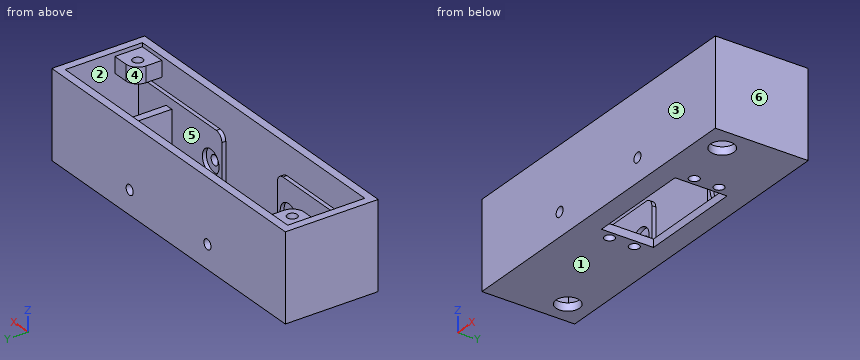
```python
from build123d import *

# Parameters (mm, degrees)
SKETCH1_W                      = 127
SKETCH1_H                      = 31.115
BOSS_EXTRUDE1_DEPTH            = 3.175
CUT_EXTRUDE1_REACH             = 5.175
SKETCH2_R                      = 2
SKETCH2_W                      = 42
SKETCH2_H                      = 21
SKETCH3_W                      = 133.35
SKETCH3_H                      = 37.465
SKETCH3_W_2                    = 127
SKETCH3_H_2                    = 31.115
EXTRUDE_THIN1_DEPTH            = 31.75
EXTRUDE_THIN1_DEPTH_BACK       = 3.175
SKETCH4_W                      = 47.625
SKETCH4_H                      = 1.5875
BOSS_EXTRUDE2_DEPTH            = 19.67500002
CUT_EXTRUDE2_REACH             = 5.175
SKETCH6_R                      = 4.7625
BOSS_EXTRUDE4_START            = -1.5875
BOSS_EXTRUDE4_DEPTH            = 6.35
CUT_EXTRUDE3_REACH             = 36.925
SKETCH8_R                      = 2
SKETCH9_R                      = 2
CUT_EXTRUDE4_DEPTH             = 19.7325
CUT_EXTRUDE4_DEPTH_BACK        = 19.7325
SKETCH5_W                      = 3.175
SKETCH5_H                      = 27.94
BOSS_EXTRUDE3_DEPTH            = 15.875
FILLET1_R                      = 3.175
CUT_EXTRUDE5_REACH             = 20.733
SKETCH10_R                     = 4.7625
CUT_EXTRUDE5_DIRECTION_2_REACH = 20.733


with BuildPart() as part:
    # Sketch1 → Boss-Extrude1 (new body)
    with BuildSketch(Plane.XY):
        Rectangle(SKETCH1_W, SKETCH1_H)
    extrude(amount=BOSS_EXTRUDE1_DEPTH)

    # Sketch2 → Cut-Extrude1 (cut, up to next)
    with BuildSketch(Plane.XY.offset(3.175), mode=Mode.PRIVATE) as cut_extrude1_sk1:
        with Locations((-13.2, 5)):
            Circle(SKETCH2_R)
    cut_extrude1_tool1 = extrude(cut_extrude1_sk1.sketch, amount=-CUT_EXTRUDE1_REACH, mode=Mode.PRIVATE) & part.part
    add(cut_extrude1_tool1.solids().sort_by_distance((-13.2, 5, 3.175))[0], mode=Mode.SUBTRACT)
    # Sketch2 → Cut-Extrude1 (cut, up to next)
    with BuildSketch(Plane.XY.offset(3.175), mode=Mode.PRIVATE) as cut_extrude1_sk2:
        with Locations((-13.2, -5)):
            Circle(SKETCH2_R)
    cut_extrude1_tool2 = extrude(cut_extrude1_sk2.sketch, amount=-CUT_EXTRUDE1_REACH, mode=Mode.PRIVATE) & part.part
    add(cut_extrude1_tool2.solids().sort_by_distance((-13.2, -5, 3.175))[0], mode=Mode.SUBTRACT)
    # Sketch2 → Cut-Extrude1 (cut, up to next)
    with BuildSketch(Plane.XY.offset(3.175), mode=Mode.PRIVATE) as cut_extrude1_sk3:
        with Locations((35.2, 5)):
            Circle(SKETCH2_R)
    cut_extrude1_tool3 = extrude(cut_extrude1_sk3.sketch, amount=-CUT_EXTRUDE1_REACH, mode=Mode.PRIVATE) & part.part
    add(cut_extrude1_tool3.solids().sort_by_distance((35.2, 5, 3.175))[0], mode=Mode.SUBTRACT)
    # Sketch2 → Cut-Extrude1 (cut, up to next)
    with BuildSketch(Plane.XY.offset(3.175), mode=Mode.PRIVATE) as cut_extrude1_sk4:
        with Locations((35.2, -5)):
            Circle(SKETCH2_R)
    cut_extrude1_tool4 = extrude(cut_extrude1_sk4.sketch, amount=-CUT_EXTRUDE1_REACH, mode=Mode.PRIVATE) & part.part
    add(cut_extrude1_tool4.solids().sort_by_distance((35.2, -5, 3.175))[0], mode=Mode.SUBTRACT)
    # Sketch2 → Cut-Extrude1 (cut, up to next)
    with BuildSketch(Plane.XY.offset(3.175), mode=Mode.PRIVATE) as cut_extrude1_sk5:
        with Locations((11, 0)):
            Rectangle(SKETCH2_W, SKETCH2_H)
    cut_extrude1_tool5 = extrude(cut_extrude1_sk5.sketch, amount=-CUT_EXTRUDE1_REACH, mode=Mode.PRIVATE) & part.part
    add(cut_extrude1_tool5.solids().sort_by_distance((11, 0, 3.175))[0], mode=Mode.SUBTRACT)

    # Sketch3 → Extrude-Thin1 (add, two sides)
    with BuildSketch(Plane.XY.offset(3.175)) as extrude_thin1_sk:
        Rectangle(SKETCH3_W, SKETCH3_H)
        Rectangle(SKETCH3_W_2, SKETCH3_H_2, mode=Mode.SUBTRACT)
    extrude(amount=EXTRUDE_THIN1_DEPTH)
    extrude(extrude_thin1_sk.sketch, amount=-EXTRUDE_THIN1_DEPTH_BACK)

    # Sketch4 → Boss-Extrude2 (add)
    with BuildSketch(Plane.XY.offset(3.175)):
        with Locations((-39.6875, -14.76375)):
            Rectangle(SKETCH4_W, SKETCH4_H)
        with Locations((39.6875, -14.76375)):
            Rectangle(SKETCH4_W, SKETCH4_H)
        with Locations((-39.6875, 14.76375)):
            Rectangle(SKETCH4_W, SKETCH4_H)
        with Locations((39.6875, 14.76375)):
            Rectangle(SKETCH4_W, SKETCH4_H)
    extrude(amount=BOSS_EXTRUDE2_DEPTH)

    # Sketch6 → Cut-Extrude2 (cut, up to next)
    with BuildSketch(Plane.XY.offset(3.175), mode=Mode.PRIVATE) as cut_extrude2_sk1:
        with Locations((-57.15, 9.2075)):
            Circle(SKETCH6_R)
    cut_extrude2_tool1 = extrude(cut_extrude2_sk1.sketch, amount=-CUT_EXTRUDE2_REACH, mode=Mode.PRIVATE) & part.part
    add(cut_extrude2_tool1.solids().sort_by_distance((-57.15, 9.2075, 3.175))[0], mode=Mode.SUBTRACT)
    # Sketch6 → Cut-Extrude2 (cut, up to next)
    with BuildSketch(Plane.XY.offset(3.175), mode=Mode.PRIVATE) as cut_extrude2_sk2:
        with Locations((57.15, -9.2075)):
            Circle(SKETCH6_R)
    cut_extrude2_tool2 = extrude(cut_extrude2_sk2.sketch, amount=-CUT_EXTRUDE2_REACH, mode=Mode.PRIVATE) & part.part
    add(cut_extrude2_tool2.solids().sort_by_distance((57.15, -9.2075, 3.175))[0], mode=Mode.SUBTRACT)

    # Sketch7 → Boss-Extrude4 (add)
    with BuildSketch(Plane.XY.offset(34.925).offset(BOSS_EXTRUDE4_START)):
        with BuildLine():
            Line((-63.5, 15.5575), (-63.5, 4.445))
            Line((-63.5, 4.445), (-57.15, 4.445))
            ThreePointArc((-57.15, 4.445), (-53.782403955, 5.839903955), (-52.3875, 9.2075))
            Line((-52.3875, 9.2075), (-52.3875, 15.5575))
            Line((-52.3875, 15.5575), (-63.5, 15.5575))
        make_face()
        with BuildLine():
            Line((63.5, -15.5575), (52.3875, -15.5575))
            Line((52.3875, -15.5575), (52.3875, -9.2075))
            ThreePointArc((52.3875, -9.2075), (53.782403955, -5.839903955), (57.15, -4.445))
            Line((57.15, -4.445), (63.5, -4.445))
            Line((63.5, -4.445), (63.5, -15.5575))
        make_face()
    extrude(amount=-BOSS_EXTRUDE4_DEPTH)

    # Sketch8 → Cut-Extrude3 (cut, up to next)
    with BuildSketch(Plane.XY.offset(34.925), mode=Mode.PRIVATE) as cut_extrude3_sk1:
        with Locations((-57.15, 9.2075)):
            Circle(SKETCH8_R)
    cut_extrude3_tool1 = extrude(cut_extrude3_sk1.sketch, amount=-CUT_EXTRUDE3_REACH, mode=Mode.PRIVATE) & part.part
    add(cut_extrude3_tool1.solids().sort_by_distance((-57.15, 9.2075, 34.925))[0], mode=Mode.SUBTRACT)
    # Sketch8 → Cut-Extrude3 (cut, up to next)
    with BuildSketch(Plane.XY.offset(34.925), mode=Mode.PRIVATE) as cut_extrude3_sk2:
        with Locations((57.15, -9.2075)):
            Circle(SKETCH8_R)
    cut_extrude3_tool2 = extrude(cut_extrude3_sk2.sketch, amount=-CUT_EXTRUDE3_REACH, mode=Mode.PRIVATE) & part.part
    add(cut_extrude3_tool2.solids().sort_by_distance((57.15, -9.2075, 34.925))[0], mode=Mode.SUBTRACT)

    # Sketch9 → Cut-Extrude4 (cut, two sides)
    with BuildSketch(Plane(origin=(0, 0, 0), x_dir=(1, 0, 0), z_dir=(0, 1, 0))) as cut_extrude4_sk:
        with Locations((22.225, -9.525)):
            Circle(SKETCH9_R)
        with Locations((-22.225, -9.525)):
            Circle(SKETCH9_R)
    extrude(amount=CUT_EXTRUDE4_DEPTH, mode=Mode.SUBTRACT)
    extrude(cut_extrude4_sk.sketch, amount=-CUT_EXTRUDE4_DEPTH_BACK, mode=Mode.SUBTRACT)

    # Sketch5 → Boss-Extrude3 (add)
    with BuildSketch(Plane.XY.offset(3.175)):
        with Locations((46.0375, 0)):
            Rectangle(SKETCH5_W, SKETCH5_H)
        with Locations((-46.0375, 0)):
            Rectangle(SKETCH5_W, SKETCH5_H)
    extrude(amount=BOSS_EXTRUDE3_DEPTH)

    # Fillet1
    fillet1_edges = [part.edges().sort_by_distance(p)[0] for p in [
        (15.875, 14.76375, 22.85000002),
        (-15.875, -14.76375, 22.85000002),
        (15.875, -14.76375, 22.85000002),
        (-15.875, 14.76375, 22.85000002),
    ]]
    fillet(fillet1_edges, radius=FILLET1_R)

    # Cut-Extrude5: up to this face of the body (flat: up to its plane)
    cut_extrude5_end = Plane(part.part.faces().sort_by_distance((-1.954505757, -15.5575, 24.090116644))[0])
    # Sketch10 → Cut-Extrude5 (cut, up to the picked face)
    with BuildSketch(Plane(origin=(0, 0, 0), x_dir=(1, 0, 0), z_dir=(0, 1, 0)), mode=Mode.PRIVATE) as cut_extrude5_sk1:
        with Locations((-22.225, -9.525)):
            Circle(SKETCH10_R)
    cut_extrude5_tool1 = split(extrude(cut_extrude5_sk1.sketch, amount=-CUT_EXTRUDE5_REACH, mode=Mode.PRIVATE), bisect_by=cut_extrude5_end, keep=Keep.BOTH, mode=Mode.PRIVATE)
    add(cut_extrude5_tool1.solids().sort_by_distance((-22.225, 0, 9.525))[0], mode=Mode.SUBTRACT)
    # Sketch10 → Cut-Extrude5 (cut, up to the picked face)
    with BuildSketch(Plane(origin=(0, 0, 0), x_dir=(1, 0, 0), z_dir=(0, 1, 0)), mode=Mode.PRIVATE) as cut_extrude5_sk2:
        with Locations((22.225, -9.525)):
            Circle(SKETCH10_R)
    cut_extrude5_tool2 = split(extrude(cut_extrude5_sk2.sketch, amount=-CUT_EXTRUDE5_REACH, mode=Mode.PRIVATE), bisect_by=cut_extrude5_end, keep=Keep.BOTH, mode=Mode.PRIVATE)
    add(cut_extrude5_tool2.solids().sort_by_distance((22.225, 0, 9.525))[0], mode=Mode.SUBTRACT)

    # Cut-Extrude5 direction 2: up to this face of the body (flat: up to its plane)
    cut_extrude5_direction_2_end = Plane(part.part.faces().sort_by_distance((1.954505757, 15.5575, 24.090116644))[0])
    # Sketch10 → Cut-Extrude5 direction 2 (cut, up to the picked face)
    with BuildSketch(Plane(origin=(0, 0, 0), x_dir=(1, 0, 0), z_dir=(0, 1, 0)), mode=Mode.PRIVATE) as cut_extrude5_direction_2_sk1:
        with Locations((-22.225, -9.525)):
            Circle(SKETCH10_R)
    cut_extrude5_direction_2_tool1 = split(extrude(cut_extrude5_direction_2_sk1.sketch, amount=CUT_EXTRUDE5_DIRECTION_2_REACH, mode=Mode.PRIVATE), bisect_by=cut_extrude5_direction_2_end, keep=Keep.BOTH, mode=Mode.PRIVATE)
    add(cut_extrude5_direction_2_tool1.solids().sort_by_distance((-22.225, 0, 9.525))[0], mode=Mode.SUBTRACT)
    # Sketch10 → Cut-Extrude5 direction 2 (cut, up to the picked face)
    with BuildSketch(Plane(origin=(0, 0, 0), x_dir=(1, 0, 0), z_dir=(0, 1, 0)), mode=Mode.PRIVATE) as cut_extrude5_direction_2_sk2:
        with Locations((22.225, -9.525)):
            Circle(SKETCH10_R)
    cut_extrude5_direction_2_tool2 = split(extrude(cut_extrude5_direction_2_sk2.sketch, amount=CUT_EXTRUDE5_DIRECTION_2_REACH, mode=Mode.PRIVATE), bisect_by=cut_extrude5_direction_2_end, keep=Keep.BOTH, mode=Mode.PRIVATE)
    add(cut_extrude5_direction_2_tool2.solids().sort_by_distance((22.225, 0, 9.525))[0], mode=Mode.SUBTRACT)


solid = part.part
```
Verification items for the finished model (mm, model axes). Face numbers are marked on the shaded views. A direction names the side the tool comes from. Round coordinates to 2 decimals unless told otherwise and drop trailing zeros. Order: outer loops, then holes, each group sorted by start corner. A loop starts at its lowest first (then second) coordinate and runs counter-clockwise, first axis right, second up. Notation, with made-up numbers: (47.25, -17) -> (95.25, -17) arc R29 cw to (95.25, 11) -> close; hole circle Ø7 at (21.25, 60). An arc over 180 degrees is marked (long way). Put each result on its own line as item: value. Start each with the question number.
(1) Material ranges on line 1 along X through (y, z) = (-10.5, 13) (3 decimals); line 2 along Y through (x, z) = (57.15, 29.25) (1 decimal); line 3 along Y through (x, z) = (-57.15, 29.75) (1 decimal), recorded low to high.
(2) Depth check by flat-ended pin: pin 1 Ø11 at (x, y) = (-57.15, 9.21) entering from +Z. Enter the tip coordinate at first touch or a pass-through.
(3) Section check A-A (x = 35.2). State how many separate pieces and enclosed holes the cut face has, then the cut area to 3 significant figures.
(4) Draft check along Y on the marked faces 1, 2 and 3. Enter one of: +Y half, -Y half, draft (parallel to the pull), parting line (faces both ways), or undercut.
(5) Tool access check on the marked faces 4, 5 and 6. Record the directions out of +Z, -Z, +X, -X, +Y, -Y that give a thin tool (end or side, any length) a straight path to the whole face; none if there is none.
(6) Section check C-C (y = 1.5). Enter the section's corners in (x, z) (3 decimals).
Completed:
1. line 1: x = -66.675 to -63.5, -47.625 to -44.45, 44.45 to 47.625, 63.5 to 66.675
1. line 2: y = -18.7 to -11.2, -7.2 to -4.4, 15.6 to 18.7
1. line 3: y = -18.7 to -15.6, 4.4 to 7.2, 11.2 to 18.7
2. pin 1: stops at z = 33.34
3. separate pieces: 3
3. enclosed holes: 0
3. area: 358 mm2
4. face 1: draft
4. face 2: undercut
4. face 3: -Y half
5. face 4: +Z
5. face 5: none
5. face 6: +Z, -Z, +X, +Y, -Y
6. outline: (-66.675, 0) -> (-10, 0) -> (-10, 3.175) -> (-44.45, 3.175) -> (-44.45, 19.05) -> (-47.625, 19.05) -> (-47.625, 3.175) -> (-63.5, 3.175) -> (-63.5, 34.925) -> (-66.675, 34.925) -> close; (32, 0) -> (66.675, 0) -> (66.675, 34.925) -> (63.5, 34.925) -> (63.5, 3.175) -> (47.625, 3.175) -> (47.625, 19.05) -> (44.45, 19.05) -> (44.45, 3.175) -> (32, 3.175) -> close
